Source: CAD feature listing. Evaluate the final solid. Frame: model axes, mm. A direction names the side the tool comes from. Round coordinates to 2 decimals unless told otherwise and drop trailing zeros. Loops run counter-clockwise (first coordinate to the right, second up) from the corner with the lowest first, then second, coordinate; pieces in that order, holes last.
Item 1: Section query B-B on x = -5.5. Return loops of the section in (y, z).
Item 2: Section query A-A on z = -29. Return loops of the section in (x, y), then the cut area to 3 significant figures.
Item 3: First-contact query: P1, Ø1.5, axis at x = -4.5, z = 21, coming from the +Y side; P2, Ø4, axis at x = -4.5, z = -10.5, coming from the -Y side. Flat tips, straight axial feed; report the tip coordinate or a pass-through.
Item 4: Access query for faces 1 (the cylindrical face through (2.44, 0.54, -41.62)), 2 (the flat face through (3, 0, -50)). Directions: +Z, -Z, +X, -X, +Y, -Y. A direction counts if a zero-diameter tool reaches every point of the face in a straight line with its end or side. Return the directions, or none.
Item 5: Section query C-C on x = 4.5. Return loops of the section in (y, z).
Item 6: Pull-direction query (X, two-part tool) for faces 3 (the cylindrical face through (2.44, 0.54, 41.62)), 4 (the flat face through (3, 0, 50)), 5 (the cylindrical face through (-1.38, -6.2, 0.7)); classes: released by +X, released by -X, zero draft, split by the parting line, or undercut.
Item 7: Ray query, L1, parallel to Y at x = 0, z = -35; L2, parallel to Y at x = 2, z = -44; L3, parallel to Z at x = -2, y = 0. Return the intervals inside material, ascending.
```python
from build123d import *

# Parameters (mm, degrees)
CROQUIS1_R              = 6.35
SALIENTE_EXTRUIR1_DEPTH = 50


with BuildPart() as part:
    # Croquis1 → Saliente-Extruir1 (new, symmetric)
    with BuildSketch(Plane.XY):
        Circle(CROQUIS1_R)
    extrude(amount=SALIENTE_EXTRUIR1_DEPTH, both=True)

    # Croquis3 → Taladro roscado M61 (revolve, cut)
    with BuildSketch(Plane(origin=(0, 0, 50), x_dir=(0, -1, 0), z_dir=(1, 0, 0))):
        Polygon((0, 0), (0, 18.502151548), (2.5, 17), (2.5, 0), align=None)
    taladro_roscado_m61 = revolve(axis=Axis((0, 0, 56.35), (0, 0, -1)), mode=Mode.SUBTRACT)

    # Simetría1: Taladro roscado M61 across plane
    add(taladro_roscado_m61.mirror(Plane.XY), mode=Mode.SUBTRACT)


solid = part.part
```
Data:
1. outline: (-3.17, -50) - (3.17, -50) - (3.17, 50) - (-3.17, 50) - close
2. outline: circle Ø12.7 at (0, 0)
2. area: 127 mm2
3. P1: stops at y = 5.12
3. P2: stops at y = -5.84
4. face 1: -Z
4. face 2: -Z, +X, -X, +Y, -Y
5. outline: (-4.48, -50) - (4.48, -50) - (4.48, 50) - (-4.48, 50) - close
6. face 3: undercut
6. face 4: zero draft
6. face 5: split by the parting line
7. L1: y = -6.35 to -2.5, 2.5 to 6.35
7. L2: y = -6.03 to -1.5, 1.5 to 6.03
7. L3: z = -32.7 to 32.7
